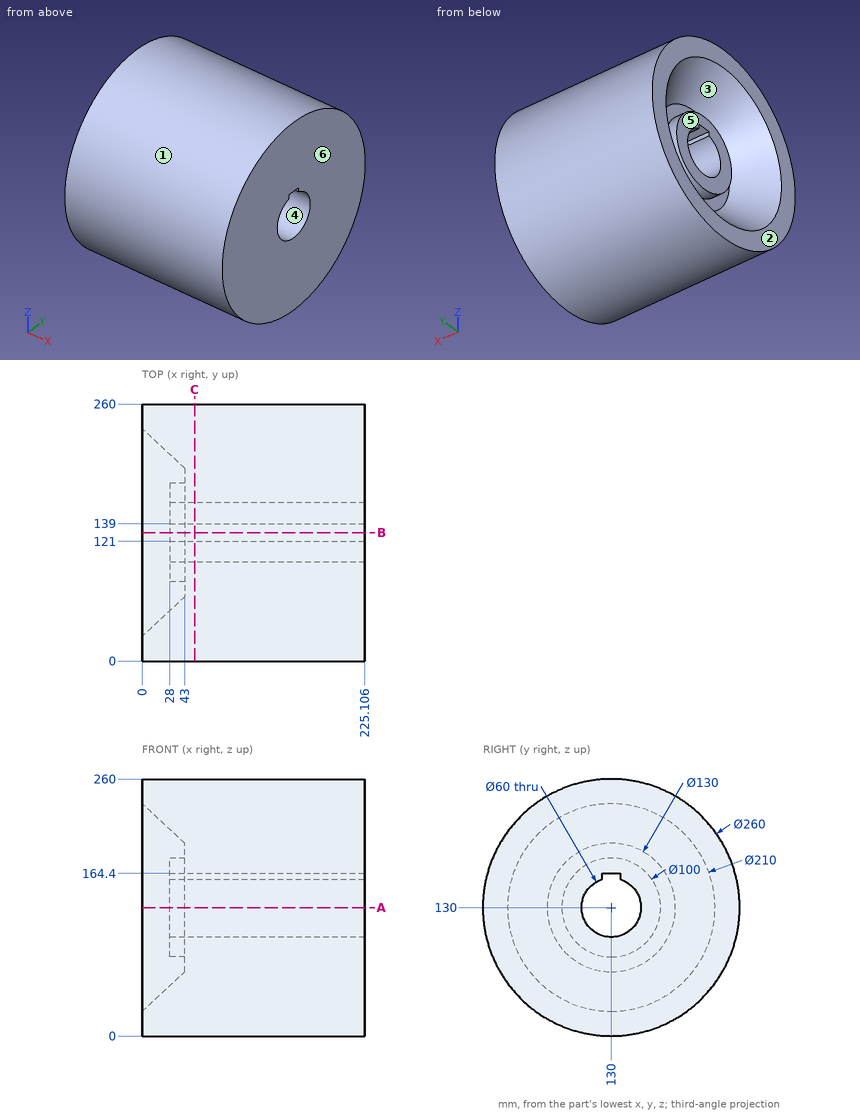
Check sheet for the drawn part. Datum: minimum x, y, z corner. Units: mm. A direction names the side the tool comes from. Round coordinates to 2 decimals unless told otherwise and drop trailing zeros. Order: outer loops, then holes, each group sorted by start corner. A loop starts at its lowest first (then second) coordinate and runs counter-clockwise, first axis right, second up.
1. Thickness scan on L1, parallel to Y at x = 105, z = 130; L2, parallel to X at y = 70, z = 117.5; L3, parallel to Z at x = 53.5, y = 136.5. Record the ranges inside material, lowest first.
Final values:
L1: y = 0 to 100, 160 to 260
L2: x = 43 to 225.11
L3: z = 0.16 to 100.71, 164.4 to 259.84
2. Section check A-A on z = 130. Record the cut outline in (x, y), then the cut area to 3 significant figures.
Final values:
outline: (0, 0) - (225.11, 0) - (225.11, 100) - (28, 100) - (28, 80) - (43, 80) - (43, 65) - (0, 25) - close; (0, 235) - (43, 195) - (43, 180) - (28, 180) - (28, 160) - (225.11, 160) - (225.11, 260) - (0, 260) - close
area: 40,900 mm2
3. Access from +Z, -Z, +X, -X, +Y, -Y to the whole of each face (thin tool, end or side, straight path). Record for the marked faces 5 and 6.
Final values:
face 5: -X
face 6: +Z, -Z, +X, +Y, -Y
4. Section check C-C on x = 53. Record the cut outline in (y, z).
Final values:
outline: circle Ø260 at (130, 130); hole (121, 158.62) arc R30 ccw (long way) to (139, 158.62) - (139, 164.4) - (121, 164.4) - close
5. Release check for a two-part mould opening along Y. For the marked faces 1, 2, 3 and 4 record: +Y half, -Y half, draft (parallel to the pull), parting line (faces both ways), or undercut.
Final values:
face 1: parting line
face 2: draft
face 3: undercut
face 4: undercut
6. Go/stop test with flat-tipped pins: P1, Ø8, axis at x = 73, y = 40.5, coming from the -Z side; P2, Ø8, axis at x = 129.5, y = 97.5, coming from the -Z side; P3, Ø3, axis at x = 97.5, z = 161, coming from the +Y side. Record where each tip stops, or that it passes through.
Final values:
P1: stops at z = 32.07
P2: stops at z = 3.16
P3: stops at y = 256.61
7. Section check B-B on y = 130. Record the cut outline in (x, z).
Final values:
outline: (0, 0) - (225.11, 0) - (225.11, 100) - (28, 100) - (28, 80) - (43, 80) - (43, 65) - (0, 25) - close; (0, 235) - (43, 195) - (43, 180) - (28, 180) - (28, 164.4) - (225.11, 164.4) - (225.11, 260) - (0, 260) - close
